from build123d import *

# Parameters (mm, degrees)
SKETCH1_W          = 698.5
SKETCH1_H          = 152.4
SKETCH1_R          = 6.985
BASE_FLANGE1_DEPTH = 9.525
FILLET1_R          = 12.7


# Sheet-metal steps are written as plain solids
with BuildPart() as part:
    # Sketch1 → Base-Flange1 (new body)
    with BuildSketch(Plane(origin=(0, 0, 0), x_dir=(1, 0, 0), z_dir=(0, 1, 0))):
        Rectangle(SKETCH1_W, SKETCH1_H)
        with Locations(Location((228.6, 38.1, 0), (0, 0, 270))):
            Circle(SKETCH1_R, mode=Mode.SUBTRACT)
        with Locations(Location((330.2, 38.1, 0), (0, 0, 270))):
            Circle(SKETCH1_R, mode=Mode.SUBTRACT)
        with Locations(Location((330.2, -38.1, 0), (0, 0, 270))):
            Circle(SKETCH1_R, mode=Mode.SUBTRACT)
        with Locations(Location((228.6, -38.1, 0), (0, 0, 270))):
            Circle(SKETCH1_R, mode=Mode.SUBTRACT)
        with Locations(Location((-228.6, -38.1, 0), (0, 0, 270))):
            Circle(SKETCH1_R, mode=Mode.SUBTRACT)
        with Locations(Location((-330.2, -38.1, 0), (0, 0, 270))):
            Circle(SKETCH1_R, mode=Mode.SUBTRACT)
        with Locations(Location((-330.2, 38.1, 0), (0, 0, 270))):
            Circle(SKETCH1_R, mode=Mode.SUBTRACT)
        with Locations(Location((-228.6, 38.1, 0), (0, 0, 270))):
            Circle(SKETCH1_R, mode=Mode.SUBTRACT)
    extrude(amount=-BASE_FLANGE1_DEPTH)

    # Fillet1
    fillet1_edges = [part.edges().sort_by_distance(p)[0] for p in [
        (349.25, -4.7625, 76.2),
        (-349.25, -4.7625, 76.2),
        (-349.25, -4.7625, -76.2),
        (349.25, -4.7625, -76.2),
    ]]
    fillet(fillet1_edges, radius=FILLET1_R)


solid = part.part
Work out the finished part from the listing and answer in its coordinate system (mm). Round coordinates to 2 decimals unless told otherwise and drop trailing zeros. Write each loop counter-clockwise with the first axis right and the second up, starting at its lowest first coordinate (ties: lowest second). Pieces come first, ordered by that corner, then holes. Notation, with made-up numbers: (83, -38.75) - (127, -38.75) arc R25 cw to (127, -14.75) - close; hole circle Ø5 at (40.5, 71.25). An arc over 180 degrees is marked (long way). Answer in a Markdown table with one row per item. Add a question column.
1. The mould has two halves that part along X. Classify faces 1 (the cylindrical face through (-337.02, -4.7, -39.61)), 2 (the cylindrical face through (345.43, -4.83, 72.58)), 3 (the flat face through (-5, 0, -1)): +X half, -X half, draft (parallel to the pull), parting line (faces both ways), or undercut.
2. A cutting plane is placed at B-B, the plane x = 330.2. Determine the outline of the cut face in (y, z) (3 decimals).
3. Find the intervals of material crossed by line 1 along Z through (x, y) = (330.2, -5) (3 decimals); line 2 along X through (y, z) = (-3, 38.1) (3 decimals), in increasing order. Write a range as from..to.
4. A cutting plane is placed at A-A, the plane z = -38.1. Determine the outline of the cut face in (x, y) (3 decimals), and give its area (3 significant figures).
5. Given pin 1 (8.5 mm diameter, centred on x = 330.2, z = 38.1, fed in from -Y), flat-ended and moving along its own axis, determine where the tip first touches the part or whether it passes through.
Worked out:
| question | item | result |
|---|---|---|
| 1 | face 1 | undercut |
| 1 | face 2 | +X half |
| 1 | face 3 | draft |
| 2 | outline | (-9.525, -76.2) - (0, -76.2) - (0, -45.085) - (-9.525, -45.085) - close; (-9.525, -31.115) - (0, -31.115) - (0, 31.115) - (-9.525, 31.115) - close; (-9.525, 45.085) - (0, 45.085) - (0, 76.2) - (-9.525, 76.2) - close |
| 3 | line 1 | -76.2..-45.085, -31.115..31.115, 45.085..76.2 |
| 3 | line 2 | -349.25..-337.185, -323.215..-235.585, -221.615..221.615, 235.585..323.215, 337.185..349.25 |
| 4 | outline | (-349.25, -9.525) - (-337.185, -9.525) - (-337.185, 0) - (-349.25, 0) - close; (-323.215, -9.525) - (-235.585, -9.525) - (-235.585, 0) - (-323.215, 0) - close; (-221.615, -9.525) - (221.615, -9.525) - (221.615, 0) - (-221.615, 0) - close; (235.585, -9.525) - (323.215, -9.525) - (323.215, 0) - (235.585, 0) - close; (337.185, -9.525) - (349.25, -9.525) - (349.25, 0) - (337.185, 0) - close |
| 4 | area | 6,120 mm^2 |
| 5 | pin 1 | through |
